```python
from build123d import *
from build123d.topology import SkipClean

# Parameters (mm, degrees)
Y_KSEKLIK_EKSTR_ZYON1_DEPTH = 60
RADYUS1_R                   = 30
IZIM4_R                     = 15
IZIM4_R_2                   = 10
Y_KSEKLIK_EKSTR_ZYON2_DEPTH = 70
IZIM5_R                     = 15
Y_KSEKLIK_EKSTR_ZYON3_DEPTH = 10
Y_KSEKLIK_EKSTR_ZYON4_START = -10
Y_KSEKLIK_EKSTR_ZYON4_DEPTH = 10
KES_EKSTR_ZYON1_START       = -10
KES_EKSTR_ZYON1_DEPTH       = 10
IZIM11_W                    = 10
IZIM11_H                    = 10
DAIRESEL_KAPLAMA3_COUNT     = 4
IZIM13_W                    = 10
IZIM13_H                    = 10
Y_KSEKLIK_EKSTR_ZYON5_DEPTH = 12.084973779
IZIM14_R                    = 10
KES_EKSTR_ZYON2_DEPTH       = 10


with BuildPart() as part:
    # Çizim2 → Yükseklik-Ekstrüzyon1 (new body)
    with BuildSketch(Plane.XY):
        Polygon((0, 0), (0, 30), (-10, 30), (-10, -10), (125, -10), (125, 0), align=None)
    extrude(amount=Y_KSEKLIK_EKSTR_ZYON1_DEPTH)

    # Radyus1
    radyus1_edges = [part.edges().sort_by_distance(p)[0] for p in [
        (125, -5, 0),
        (125, -5, 60),
    ]]
    fillet(radyus1_edges, radius=RADYUS1_R - 0.0001)  # a hair under: the kernel refuses the full size

    # Çizim4 → Yükseklik-Ekstrüzyon2 (add)
    with BuildSketch(Plane.XZ.offset(10)):
        with Locations((95, 30)):
            Circle(IZIM4_R)
        with Locations((95, 30)):
            Circle(IZIM4_R_2, mode=Mode.SUBTRACT)
    extrude(amount=-Y_KSEKLIK_EKSTR_ZYON2_DEPTH)

    # Çizim5 → Yükseklik-Ekstrüzyon3 (add)
    with BuildSketch(Plane(origin=(0, 60, 0), x_dir=(1, 0, 0), z_dir=(0, 1, 0))):
        with Locations((95, -30)):
            Circle(IZIM5_R)
    extrude(amount=Y_KSEKLIK_EKSTR_ZYON3_DEPTH)

    # Çizim7 → Yükseklik-Ekstrüzyon4 (add)
    with BuildSketch(Plane(origin=(0, 30, 0), x_dir=(1, 0, 0), z_dir=(0, 1, 0)).offset(Y_KSEKLIK_EKSTR_ZYON4_START)):
        with BuildLine():
            Line((95, 45), (30, 45))
            ThreePointArc((30, 45), (1.715728753, 33.284271247), (-10, 5))
            Line((-10, 5), (-10, -65))
            ThreePointArc((-10, -65), (1.715728753, -93.284271247), (30, -105))
            Line((30, -105), (94.99998957, -105))
            ThreePointArc((94.99998957, -105), (170, -30.000005215), (95, 45))
        make_face()
        with BuildLine():
            Line((80, -95), (30, -95))
            ThreePointArc((30, -95), (8.786796564, -86.213203436), (0, -65))
            ThreePointArc((0, -65), (8.786796564, -43.786796564), (30, -35))
            Line((30, -35), (80.857864376, -35))
            ThreePointArc((80.857864376, -35), (80, -30), (80.857864376, -25))
            Line((80.857864376, -25), (30, -25))
            ThreePointArc((30, -25), (0, 5), (30, 35))
            Line((30, 35), (80, 35))
            ThreePointArc((80, 35), (87.071067812, 32.071067812), (90, 25))
            Line((90, 25), (90, -15.857864376))
            ThreePointArc((90, -15.857864376), (95, -15), (100, -15.857864376))
            Line((100, -15.857864376), (100, 22.915026221))
            ThreePointArc((100, 22.915026221), (103.969773108, 30.892266573), (112.727272727, 32.53594008))
            ThreePointArc((112.727272727, 32.53594008), (140.961940777, 15.961940777), (157.53594008, -12.272727273))
            ThreePointArc((157.53594008, -12.272727273), (155.892266573, -21.030226892), (147.915026221, -25))
            Line((147.915026221, -25), (109.142135624, -25))
            ThreePointArc((109.142135624, -25), (110, -30), (109.142135624, -35))
            Line((109.142135624, -35), (147.915026221, -35))
            ThreePointArc((147.915026221, -35), (155.892266573, -38.969773108), (157.53594008, -47.727272727))
            ThreePointArc((157.53594008, -47.727272727), (140.961940777, -75.961940777), (112.727272727, -92.53594008))
            ThreePointArc((112.727272727, -92.53594008), (103.969773108, -90.892266573), (100, -82.915026221))
            Line((100, -82.915026221), (100, -44.142135624))
            ThreePointArc((100, -44.142135624), (95, -45), (90, -44.142135624))
            Line((90, -44.142135624), (90, -85))
            ThreePointArc((90, -85), (87.071067812, -92.071067812), (80, -95))
        make_face(mode=Mode.SUBTRACT)
    extrude(amount=Y_KSEKLIK_EKSTR_ZYON4_DEPTH)

    # Çizim8 → Kes-Ekstrüzyon1 (cut)
    with SkipClean():  # the faces are left unmerged after this step: merging them gives an invalid solid
        with BuildSketch(Plane(origin=(0, 30, 0), x_dir=(1, 0, 0), z_dir=(0, 1, 0)).offset(KES_EKSTR_ZYON1_START)):
            with BuildLine():
                Line((30, -25), (80.857864376, -25))
                ThreePointArc((80.857864376, -25), (80, -30), (80.857864376, -35))
                Line((80.857864376, -35), (30, -35))
                Line((30, -35), (30, -25))
            make_face()
            with BuildLine():
                Line((147.915026221, -25), (147.915026221, -35))
                Line((147.915026221, -35), (109.142135624, -35))
                ThreePointArc((109.142135624, -35), (110, -30), (109.142135624, -25))
                Line((109.142135624, -25), (147.915026221, -25))
            make_face()
            with BuildLine():
                Line((100, 22.915026221), (90, 22.915026221))
                Line((90, 22.915026221), (90, -15.857864376))
                ThreePointArc((90, -15.857864376), (95, -15), (100, -15.857864376))
                Line((100, -15.857864376), (100, 22.915026221))
            make_face()
            with BuildLine():
                Line((100, -82.915026221), (90, -82.915026221))
                Line((90, -82.915026221), (90, -44.142135624))
                ThreePointArc((90, -44.142135624), (95, -45), (100, -44.142135624))
                Line((100, -44.142135624), (100, -82.915026221))
            make_face()
        extrude(amount=KES_EKSTR_ZYON1_DEPTH, mode=Mode.SUBTRACT)
    add(part.part.scale(1), mode=Mode.REPLACE)  # the faces are merged on a copy

    # Süpür1: sweep along a path in Çizim10
    with BuildLine(Plane.XY.offset(30)) as s_p_r1_path:
        Line((95, 70), (115, 70))
        ThreePointArc((115, 70), (125.606601718, 65.606601718), (130, 55))
        Line((130, 55), (130, 45))
        ThreePointArc((130, 45), (134.393398282, 34.393398282), (145, 30))
        Line((145, 30), (147.915026221, 30))
    # Çizim11 → Süpür1 (sweep)
    with BuildSketch(Plane.ZY.offset(-147.915026221)):
        with Locations((30, 25)):
            Rectangle(IZIM11_W, IZIM11_H)
    s_p_r1 = sweep(path=s_p_r1_path.line)

    # Dairesel Kaplama3: Süpür1 ×4 about axis
    dairesel_kaplama3_axis = Axis((95, 0, 30), (0, 1, 0))
    for i in range(1, DAIRESEL_KAPLAMA3_COUNT):
        add(s_p_r1.rotate(dairesel_kaplama3_axis, i * 360 / DAIRESEL_KAPLAMA3_COUNT))

    # Çizim13 → Yükseklik-Ekstrüzyon5 (add)
    with BuildSketch(Plane(origin=(30, 0, 0), x_dir=(0, 0, -1), z_dir=(1, 0, 0))):
        with Locations((-30, 25)):
            Rectangle(IZIM13_W, IZIM13_H)
    extrude(amount=Y_KSEKLIK_EKSTR_ZYON5_DEPTH)

    # Çizim14 → Kes-Ekstrüzyon2 (cut)
    with BuildSketch(Plane.XZ.offset(10)):
        with Locations((95, 30)):
            Circle(IZIM14_R)
    extrude(amount=-KES_EKSTR_ZYON2_DEPTH, mode=Mode.SUBTRACT)


solid = part.part
```
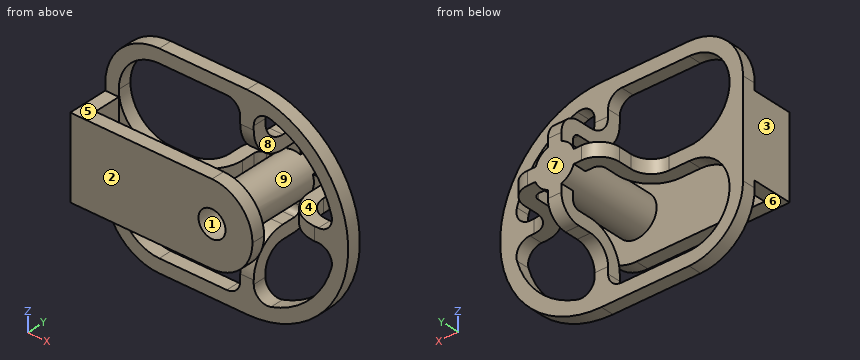
The model under review builds one solid part; all positions refer to its coordinate system, in mm. Face numbers are marked on the shaded views. A direction names the side the tool comes from. Round coordinates to 2 decimals unless told otherwise and drop trailing zeros. Order: outer loops, then holes, each group sorted by start corner. A loop starts at its lowest first (then second) coordinate and runs counter-clockwise, first axis right, second up.
(1) Mouldability with a two-part tool opening along X and no side actions: class the marked faces 1, 2, 3 and 4 as released by +X, released by -X, zero draft, split by the parting line, or undercut.
Working result:
face 1: undercut
face 2: zero draft
face 3: released by -X
face 4: undercut
(2) Take a section at C-C, the plane y = 38. State the section outline as (x, z) points.
Working result:
outline: (58.27, 25) - (69, 25) - (69, 35) - (58.27, 35) - close; circle Ø30 at (95, 30); (90, -6.73) - (100, -6.73) - (100, 4) - (90, 4) - close; (90, 56) - (100, 56) - (100, 66.73) - (90, 66.73) - close; (121, 25) - (131.73, 25) - (131.73, 35) - (121, 35) - close; hole circle Ø20 at (95, 30)
(3) Take a section at D-D, the plane x = 4.5. State the section outline as (y, z) points.
Working result:
outline: (-10, 0) - (0, 0) - (0, 60) - (-10, 60) - close; (20, -35.82) - (30, -35.82) - (30, -20.8) - (20, -20.8) - close; (20, 10.8) - (30, 10.8) - (30, 49.2) - (20, 49.2) - close; (20, 80.8) - (30, 80.8) - (30, 95.82) - (20, 95.82) - close
(4) Wall thickness on L1, parallel to Z at x = 98, y = 28.5; L2, parallel to Z at x = 92, y = 44; L3, parallel to Z at x = 20.5, y = -6: over which ranges is each line inside the solid? List them lowest first.
Working result:
L1: z = -44.94 to -1.22, 15.3 to 20.46, 39.54 to 44.7, 61.22 to 104.94
L2: z = -5.03 to 4.98, 15.3 to 20.46, 39.54 to 44.7, 55.02 to 65.03
L3: z = 0 to 60
(5) Take a section at B-B, the plane y = 6.5. State the section outline as (x, z) points.
Working result:
outline: (-10, 0) - (0, 0) - (0, 60) - (-10, 60) - close; circle Ø30 at (95, 30); hole circle Ø20 at (95, 30)
(6) For P1, Ø11, axis at y = 48, z = 31, coming from the +X side; P2, Ø12, axis at x = 95, z = 30, coming from the -Y side; P3, Ø11.5, axis at x = 135, y = 42, coming from the +Z side, all flat-tipped, find the tip position at first contact; note any pin that passes through.
Working result:
P1: stops at x = 130.21
P2: stops at y = 60
P3: stops at z = 35
(7) Tool access review of the marked faces 5, 6, 7, 8 and 9: name each direction out of +Z, -Z, +X, -X, +Y, -Y from which nothing blocks a thin tool from reaching the whole face with its end or side.
Working result:
face 5: +Z, +X, -X, -Y
face 6: -Z, +X, -X, -Y
face 7: +Z, -Z, +X, -X, +Y
face 8: +Y
face 9: none
(8) Take a section at A-A, the plane x = 37.5. State the section outline as (y, z) points, plus the area to 3 significant figures.
Working result:
outline: (-10, 0) - (0, 0) - (0, 60) - (-10, 60) - close; (20, -45) - (30, -45) - (30, -35) - (20, -35) - close; (20, 25) - (30, 25) - (30, 35) - (20, 35) - close; (20, 95) - (30, 95) - (30, 105) - (20, 105) - close
area: 900 mm2
